Build history of the part. All positions in model axes, mm. Face numbers are marked on the shaded views. A direction names the side the tool comes from. Give positions to 0.01 mm unless a question says otherwise; leave off trailing zeros. Order: outer loops, then holes, each group sorted by start corner. A loop starts at its lowest first (then second) coordinate and runs counter-clockwise, first axis right, second up. Notation, with made-up numbers: M 33.5,80 L 44.5,80 A21 cw 44.5,97 Z; hole C 65.5,-27.5 d4. An arc over 180 degrees is marked long. Use CSV: the item, a comma, the result in double quotes. Start each with the question number.
Item 1: Pin check, flat tips, straight feed: P1, Ø1, axis at x = 6, z = 6, coming from the -Y side; P2, Ø2, axis at y = 200, z = 1.5, coming from the -X side; P3, Ø11, axis at y = 252, z = -4.5, coming from the -X side; P4, Ø5, axis at x = 14.5, y = 227.5, coming from the +Z side. Stop position of each tip, or through.
Item 2: Which spindle directions (+Z, -Z, +X, -X, +Y, -Y) get a long thin tool onto all of the face, cutting with end or side? Do the marked faces 4, 5, 6, 7 and 8. Say none if no direction does.
Item 3: Band-saw the part on A-A on y = 225. Write the cut outline in (x, z).
Item 4: Two-plate mould, pull along X, no slides. Class the marked faces 1, 2 and 3: pulls with the +X half, pulls with the -X half, needs draft (parallel to the pull), parting line crosses it, or undercut.
Item 5: Band-saw the part on B-B on z = -15.5. Write the cut outline in (x, y), plus the area to 3 significant figures.
Item 6: Band-saw the part on C-C on x = 0. Give the number of separate pieces and of enclosed holes in the cut face, plus the area to 3 significant figures.
Item 7: Band-saw the part on D-D on y = 250. Write the cut outline in (x, z).
Item 8: Wall check: line 1 along Y through (x, z) = (0, 6.25); line 2 along Z through (x, y) = (7, 247); line 3 along X through (y, z) = (190, -14). Give the ranges that are in metal, low to high.
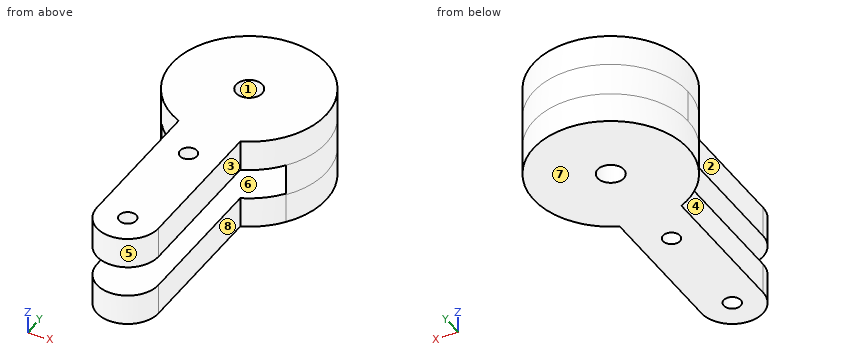
from build123d import *

# Parameters (mm, degrees)
SKETCH2_R           = 2.75
SKETCH2_R_2         = 4.25
BOSS_EXTRUDE1_DEPTH = 10
BOSS_EXTRUDE2_START = 10.4
BOSS_EXTRUDE2_DEPTH = 10.4
BOSS_EXTRUDE3_START = 10.4
SKETCH4_R           = 2.75
SKETCH4_R_2         = 4.25
BOSS_EXTRUDE3_DEPTH = 10.4
SKETCH5_R           = 4.25
BOSS_EXTRUDE4_DEPTH = 0.4
CUT_EXTRUDE2_DEPTH  = 0.4
CUT_EXTRUDE3_DEPTH  = 0.4


with BuildPart() as part:
    # Sketch2 → Boss-Extrude1 (new body)
    with BuildSketch(Plane.XY):
        with BuildLine():
            ThreePointArc((10, 237.087122), (0, 285), (-10, 237.087122))
            Line((-10, 237.087122), (-10, 190))
            ThreePointArc((-10, 190), (0, 180), (10, 190))
            Line((10, 190), (10, 237.087122))
        make_face()
        with Locations((0, 225)):
            Circle(SKETCH2_R, mode=Mode.SUBTRACT)
        with Locations((0, 260)):
            Circle(SKETCH2_R_2, mode=Mode.SUBTRACT)
        with Locations((0, 190)):
            Circle(SKETCH2_R, mode=Mode.SUBTRACT)
    extrude(amount=BOSS_EXTRUDE1_DEPTH)

    # Sketch3 → Boss-Extrude2 (add)
    with BuildSketch(Plane(origin=(0, 0, 0), x_dir=(-1, 0, 0), z_dir=(0, 0, -1)).offset(BOSS_EXTRUDE2_START)):
        with BuildLine():
            Line((-20.2, 245.270438), (-20.2, 260))
            ThreePointArc((-20.2, 260), (0, 280.2), (20.2, 260))
            Line((20.2, 260), (20.2, 245.270438))
            ThreePointArc((20.2, 245.270438), (23.769729, 252.254033), (25, 260))
            ThreePointArc((25, 260), (-7.745967, 283.769729), (-20.2, 245.270438))
        make_face()
    extrude(amount=-BOSS_EXTRUDE2_DEPTH)

    # Sketch4 → Boss-Extrude3 (add)
    # profile 1 of 2: a face of its own
    with BuildSketch(Plane(origin=(0, 0, -10.4), x_dir=(-1, 0, 0), z_dir=(0, 0, -1)).offset(BOSS_EXTRUDE3_START)):
        with BuildLine():
            Line((10, 190), (10, 237.087122))
            ThreePointArc((10, 237.087122), (15.644541, 240.500043), (20.2, 245.270438))
            Line((20.2, 245.270438), (20.2, 260))
            ThreePointArc((20.2, 260), (0, 280.2), (-20.2, 260))
            Line((-20.2, 260), (-20.2, 245.270438))
            ThreePointArc((-20.2, 245.270438), (-15.644541, 240.500043), (-10, 237.087122))
            Line((-10, 237.087122), (-10, 190))
            ThreePointArc((-10, 190), (0, 180), (10, 190))
        make_face()
        with Locations(Location((0, 190, 0), (0, 0, 180))):
            Circle(SKETCH4_R, mode=Mode.SUBTRACT)
        with Locations(Location((0, 225, 0), (0, 0, 180))):
            Circle(SKETCH4_R, mode=Mode.SUBTRACT)
        with Locations(Location((0, 260, 0), (0, 0, 180))):
            Circle(SKETCH4_R_2, mode=Mode.SUBTRACT)
    # profile 2 of 2: a face of its own
    with BuildSketch(Plane(origin=(0, 0, -10.4), x_dir=(-1, 0, 0), z_dir=(0, 0, -1)).offset(BOSS_EXTRUDE3_START)):
        with BuildLine():
            Line((-20.2, 245.270438), (-20.2, 260))
            ThreePointArc((-20.2, 260), (0, 280.2), (20.2, 260))
            Line((20.2, 260), (20.2, 245.270438))
            ThreePointArc((20.2, 245.270438), (0, 285), (-20.2, 245.270438))
        make_face()
    extrude(amount=-BOSS_EXTRUDE3_DEPTH)

    # Sketch5 → Boss-Extrude4 (add)
    with BuildSketch(Plane.XY.offset(-10.4)):
        with BuildLine():
            Line((-20.2, 260), (-20.2, 245.270438))
            ThreePointArc((-20.2, 245.270438), (-15.644541, 240.500043), (-10, 237.087122))
            Line((-10, 237.087122), (-10, 190))
            ThreePointArc((-10, 190), (0, 180), (10, 190))
            Line((10, 190), (10, 237.087122))
            ThreePointArc((10, 237.087122), (15.644541, 240.500043), (20.2, 245.270438))
            Line((20.2, 245.270438), (20.2, 260))
            ThreePointArc((20.2, 260), (0, 280.2), (-20.2, 260))
        make_face()
        with Locations((0, 260)):
            Circle(SKETCH5_R, mode=Mode.SUBTRACT)
    extrude(amount=BOSS_EXTRUDE4_DEPTH)

    # Sketch7 → Cut-Extrude2 (cut)
    with BuildSketch(Plane(origin=(0, 0, -20.8), x_dir=(-1, 0, 0), z_dir=(0, 0, -1))):
        with BuildLine():
            Line((-10, 237.087122), (-10, 190))
            ThreePointArc((-10, 190), (0, 180), (10, 190))
            Line((10, 190), (10, 237.087122))
            ThreePointArc((10, 237.087122), (0, 285), (-10, 237.087122))
        make_face()
    extrude(amount=-CUT_EXTRUDE2_DEPTH, mode=Mode.SUBTRACT)

    # Sketch8 → Cut-Extrude3 (cut)
    with BuildSketch(Plane(origin=(0, 0, -20.4), x_dir=(-1, 0, 0), z_dir=(0, 0, -1))):
        with BuildLine():
            Line((-10, 237.087122), (-10, 190))
            ThreePointArc((-10, 190), (0, 180), (10, 190))
            Line((10, 190), (10, 237.087122))
            ThreePointArc((10, 237.087122), (0, 285), (-10, 237.087122))
        make_face()
    extrude(amount=-CUT_EXTRUDE3_DEPTH, mode=Mode.SUBTRACT)


solid = part.part
Model answer:
1,P1,"stops at y = 181.65"
1,P2,"stops at x = -10"
1,P3,"stops at x = -24.87"
1,P4,"passes through"
2,face 4,"+Z, -Z, -X, -Y"
2,face 5,"+Z, -Z, -Y"
2,face 6,"-Y"
2,face 7,"-Z, +X, -X, +Y, -Y"
2,face 8,"+Z, -Z, +X, -Y"
3,outline,"M -10,-20 L -2.75,-20 L -2.75,-10.4 L 2.75,-10.4 L 2.75,-20 L 10,-20 L 10,-10 L -10,-10 Z; M -10,0 L -2.75,0 L -2.75,10 L -10,10 Z; M 2.75,0 L 10,0 L 10,10 L 2.75,10 Z"
4,face 1,"undercut"
4,face 2,"pulls with the -X half"
4,face 3,"pulls with the +X half"
5,outline,"M -20.2,245.27 A25 ccw -10,237.09 L -10,190 A10 ccw 10,190 L 10,237.09 A25 ccw 20.2,245.27 A25 ccw long Z; hole C 0,260 d8.5; hole C 0,190 d5.5; hole C 0,225 d5.5"
5,area,"2,930 mm^2"
6,separate pieces,"5"
6,enclosed holes,"0"
6,area,"1,760 mm^2"
7,outline,"M -22.91,-20 L 22.91,-20 L 22.91,10 L -22.91,10 Z; hole M -20.2,-10 L 20.2,-10 L 20.2,0 L -20.2,0 Z"
8,line 1,"y = 180 to 187.25, 192.75 to 222.25, 227.75 to 255.75, 264.25 to 285"
8,line 2,"z = -20 to -10, 0 to 10"
8,line 3,"x = -10 to -2.75, 2.75 to 10"
